Work out the finished part from the listing and answer in its coordinate system (mm). Face numbers are marked on the shaded views. A direction names the side the tool comes from. Round coordinates to 2 decimals unless told otherwise and drop trailing zeros. Order: outer loops, then holes, each group sorted by start corner. A loop starts at its lowest first (then second) coordinate and runs counter-clockwise, first axis right, second up. Notation, with made-up numbers: M 53,67.25 L 95,67.25 A15 cw 95,73.25 Z; hole C 37.5,-11 d5. An arc over 180 degrees is marked long. Answer as a JSON object with one key per item and string values. Group by question number.
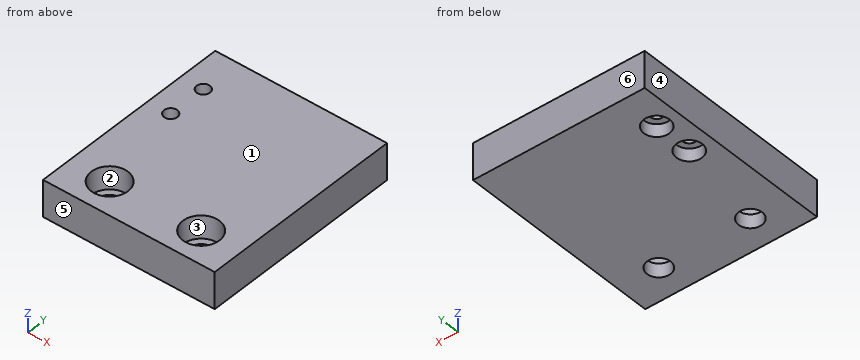
from build123d import *

# Parameters (mm, degrees)
SKETCH1_W                                        = 47.6504
SKETCH1_H                                        = 56.4388
BOSS_EXTRUDE1_DEPTH                              = 10.16
CBORE_FOR_1_4_BUTTON_HEAD_CAP_SCREW1_D           = 6.5278
CBORE_FOR_1_4_BUTTON_HEAD_CAP_SCREW1_CBORE_D     = 10.16
CBORE_FOR_1_4_BUTTON_HEAD_CAP_SCREW1_CBORE_DEPTH = 6.35
CBORE_FOR_6_SOCKET_HEAD_CAP_SCREW1_D             = 3.6576
CBORE_FOR_6_SOCKET_HEAD_CAP_SCREW1_CBORE_D       = 7.14502
CBORE_FOR_6_SOCKET_HEAD_CAP_SCREW1_CBORE_DEPTH   = 3.5052


with BuildPart() as part:
    # Sketch1 → Boss-Extrude1 (new body)
    with BuildSketch(Plane.XY):
        with Locations((23.8252, 28.2194)):
            Rectangle(SKETCH1_W, SKETCH1_H)
    extrude(amount=BOSS_EXTRUDE1_DEPTH)

    # CBORE for 1/4 Button Head Cap Screw1 (through all)
    with Locations(Plane.XY.offset(10.16)):
        with Locations((36.5125, 8.7122), (11.1125, 8.7122)):
            CounterBoreHole(CBORE_FOR_1_4_BUTTON_HEAD_CAP_SCREW1_D / 2, CBORE_FOR_1_4_BUTTON_HEAD_CAP_SCREW1_CBORE_D / 2, CBORE_FOR_1_4_BUTTON_HEAD_CAP_SCREW1_CBORE_DEPTH)

    # CBORE for #6 Socket Head Cap Screw1 (through all)
    with Locations(Plane(origin=(0, 0, 0), x_dir=(-1, 0, 0), z_dir=(0, 0, -1))):
        with Locations((-6.35, 34.3408), (-6.35, 45.0088)):
            CounterBoreHole(CBORE_FOR_6_SOCKET_HEAD_CAP_SCREW1_D / 2, CBORE_FOR_6_SOCKET_HEAD_CAP_SCREW1_CBORE_D / 2, CBORE_FOR_6_SOCKET_HEAD_CAP_SCREW1_CBORE_DEPTH)


solid = part.part
Item 1: Each of these flat-tipped pins is pushed along its axis until it touches: pin 1 (4.5 mm diameter, centred on x = 6.35, y = 34.34, fed in from -Z); pin 2 (7.5 mm diameter, centred on x = 36.51, y = 8.71, fed in from +Z). Where does it stop, or does it pass through?
Item 2: Find section B-B (x = 37). Give the vertices of the cut face in (y, z), and give its area (3 significant figures).
Item 3: Find section A-A (z = 7.75). Give the vertices of the cut face in (x, y).
Item 4: The mould has two halves that part along Y. Classify the marked faces 3, 4, 5 and 6: +Y half, -Y half, draft (parallel to the pull), parting line (faces both ways), or undercut.
Item 5: A tool of negligible diameter and unlimited length cuts with its end or side. For the marked faces 1 and 2, from which of +Z, -Z, +X, -X, +Y, -Y can it reach the whole face along a straight path? Write none if from no direction.
Item 6: Consider L1, parallel to X at y = 11.5, z = 8; L2, parallel to X at y = 10.5, z = 9.5; L3, parallel to X at y = 44, z = 3. Determine where each line is inside the solid, lowest interval first.
Responses:
{
 "1": {"pin 1": "stops at z = 3.51", "pin 2": "stops at z = 3.81"},
 "2": {"outline": "M 0,0 L 5.48,0 L 5.48,3.81 L 3.66,3.81 L 3.66,10.16 L 0,10.16 Z; M 11.94,0 L 56.44,0 L 56.44,10.16 L 13.77,10.16 L 13.77,3.81 L 11.94,3.81 Z", "area": "485 mm^2"},
 "3": {"outline": "M 0,0 L 47.65,0 L 47.65,56.44 L 0,56.44 Z; hole C 6.35,34.34 d3.66; hole C 6.35,45.01 d3.66; hole C 11.11,8.71 d10.16; hole C 36.51,8.71 d10.16"},
 "4": {"face 3": "undercut", "face 4": "draft", "face 5": "-Y half", "face 6": "+Y half"},
 "5": {"face 1": "+Z, +X, -X, +Y, -Y", "face 2": "+Z"},
 "6": {"L1": "x = 0 to 6.87, 15.36 to 32.27, 40.76 to 47.65", "L2": "x = 0 to 6.36, 15.87 to 31.76, 41.27 to 47.65", "L3": "x = 0 to 2.92, 9.78 to 47.65"}
}
